The listing builds one solid part. Answer for the finished solid, in the listing's coordinates (mm). Round coordinates to 2 decimals unless told otherwise and drop trailing zeros. Loops run counter-clockwise (first coordinate to the right, second up) from the corner with the lowest first, then second, coordinate; pieces in that order, holes last. Notation, with made-up numbers: (13.25, 49.25) - (44.25, 49.25) arc R15 cw to (44.25, 62.25) - close; hole circle Ø2 at (37, -26.5). An arc over 180 degrees is marked (long way). Write item = value, one per line. Start each with the question number.
1) Section C-C, the plane y = 17.5 is taken. Determine the outline of the cut face in (x, z), and give its area (3 significant figures).
2) Section A-A, the plane x = 12.7 is taken. Determine the outline of the cut face in (y, z).
3) Given pin 1 Ø4 at (x, z) = (14.5, 3.5) entering from -Y, flat-ended and moving along its own axis, determine where the tip first touches the part or whether it passes through.
4) A straight line is drawn through the part: line 1 along Z through (x, y) = (5.25, 12.7). Find the intervals that lie inside material, in ascending order.
5) For a pull along Y with two mould halves and no side action, classify faces 1 (the cylindrical face through (10.213, 12.809, 5.547)), 2 (the flat face through (15.34, 0, 12.52)), 3 (the cylindrical face through (20.01, 15, 11.75)), 4 (the cylindrical face through (10.213, 19.853, 12.809)) as released by +Y, released by -Y, zero draft, split by the parting line, or undercut.
from build123d import *

# Parameters (mm, degrees)
F0_W     = 25.4
F0_H     = 25.4
F1_DEPTH = 25.4
F2_R     = 2.4892
F3_DEPTH = 25.4
F4_R     = 2.4892
F5_DEPTH = 25.4
F6_R     = 2.4892
F7_DEPTH = 25.4


with BuildPart() as f1:
    # F0 (on Top) → F1 (new body)
    with BuildSketch(Plane.XY):
        with Locations((12.7, 12.7)):
            Rectangle(F0_W, F0_H)
    extrude(amount=F1_DEPTH)

    # F2 (on face) → F3 (cut)
    with BuildSketch(Plane.XY.offset(25.4)):
        with Locations((12.7, 12.7)):
            Circle(F2_R)
    extrude(amount=-F3_DEPTH, mode=Mode.SUBTRACT)

    # F4 (on face) → F5 (cut)
    with BuildSketch(Plane.YZ.offset(25.4)):
        with Locations((12.7, 12.7)):
            Circle(F4_R)
    extrude(amount=-F5_DEPTH, mode=Mode.SUBTRACT)

    # F6 (on face) → F7 (cut)
    with BuildSketch(Plane.XZ):
        with Locations((12.7, 12.7)):
            Circle(F6_R)
    extrude(amount=-F7_DEPTH, mode=Mode.SUBTRACT)


solid = f1.part
Geometry check:
q1.outline = (0, 0) - (25.4, 0) - (25.4, 25.4) - (0, 25.4) - close; hole circle Ø4.98 at (12.7, 12.7)
q1.area = 626 mm2
q2.outline = (0, 0) - (10.21, 0) - (10.21, 10.21) - (0, 10.21) - close; (0, 15.19) - (10.21, 15.19) - (10.21, 25.4) - (0, 25.4) - close; (15.19, 0) - (25.4, 0) - (25.4, 10.21) - (15.19, 10.21) - close; (15.19, 15.19) - (25.4, 15.19) - (25.4, 25.4) - (15.19, 25.4) - close
q3.pin_1 = 0
q4.line_1 = 0 to 10.21, 15.19 to 25.4
q5.face_1 = undercut
q5.face_2 = released by -Y
q5.face_3 = undercut
q5.face_4 = zero draft
